from build123d import *

# Parameters (mm, degrees)
PAD_DEPTH       = 2
CHAMFER_SIZE    = 1
FILLET_R        = 1
SKETCH002_W     = 1.2
SKETCH002_H     = 3
PAD001_DEPTH    = 4.5
CHAMFER001_SIZE = 0.2


with BuildPart() as part:
    # Sketch → Pad (new body)
    with BuildSketch(Plane.XY):
        Polygon((17.999992, 0), (17.999992, 10.3923), (8.999996, 15.58845), (0, 10.3923), (0, 0), (8.999996, -5.19615), align=None)
    extrude(amount=PAD_DEPTH)

    # Chamfer
    chamfer_edges = [part.edges().sort_by_distance(p)[0] for p in [
        (13.499994, -2.598075, 2),
        (4.499998, -2.598075, 2),
        (17.999992, 5.19615, 2),
        (13.499994, 12.990375, 2),
        (0, 5.19615, 2),
        (4.499998, 12.990375, 2),
    ]]
    chamfer(chamfer_edges, length=CHAMFER_SIZE)

    # Fillet
    fillet_edges = [part.edges().sort_by_distance(p)[0] for p in [
        (13.499994, 12.990375, 1),
        (13.499994, -2.598075, 1),
        (17.999992, 5.19615, 1),
        (4.499998, -2.598075, 1),
        (0, 5.19615, 1),
        (4.499998, 12.990375, 1),
    ]]
    fillet(fillet_edges, radius=FILLET_R)

    # Sketch002 → Pad001 (join)
    with BuildSketch(Plane(origin=(0, 0, 0.01), x_dir=(1, 0, 0), z_dir=(0, 0, -1))):
        with Locations((6.149996, -5.19615)):
            Rectangle(SKETCH002_W, SKETCH002_H)
        with Locations((11.849996, -5.19615)):
            Rectangle(SKETCH002_W, SKETCH002_H)
    extrude(amount=PAD001_DEPTH)

    # Chamfer001
    chamfer001_edges = [part.edges().sort_by_distance(p)[0] for p in [
        (11.849996, 3.69615, -4.49),
        (11.249996, 5.19615, -4.49),
        (11.849996, 6.69615, -4.49),
        (12.449996, 5.19615, -4.49),
        (11.249996, 3.69615, -2.245),
        (11.249996, 6.69615, -2.245),
        (12.449996, 3.69615, -2.245),
        (12.449996, 6.69615, -2.245),
        (5.549996, 5.19615, -4.49),
        (6.149996, 3.69615, -4.49),
        (6.749996, 5.19615, -4.49),
        (6.149996, 6.69615, -4.49),
        (5.549996, 3.69615, -2.245),
        (6.749996, 3.69615, -2.245),
        (5.549996, 6.69615, -2.245),
        (6.749996, 6.69615, -2.245),
    ]]
    chamfer(chamfer001_edges, length=CHAMFER001_SIZE)


solid = part.part
Verification items for the finished model (mm, model axes). A direction names the side the tool comes from. Give positions to 0.01 mm unless a question says otherwise; leave off trailing zeros. Loops run counter-clockwise (first coordinate to the right, second up) from the corner with the lowest first, then second, coordinate; pieces in that order, holes last.
1) Sectioned sample at D-D, the plane z = 1. Enter the section's corners in (x, y).
2) Draft check along X on faces 6 (the flat face through (6, 5, -4.49)), 7 (the flat face through (5.55, 5, -2)), 8 (the flat face through (6.75, 5, -2)), 9 (the flat face through (13.563, 12.954, 0.289)). Enter one of: pulls with the +X half, pulls with the -X half, needs draft (parallel to the pull), parting line crosses it, or undercut.
3) Depth check by flat-ended pin: pin 1 Ø0.8 at (y, z) = (5, -2.5) entering from -X; pin 2 Ø6 at (x, y) = (13.5, 0.5) entering from -Z; pin 3 Ø0.9 at (x, z) = (6, -3) entering from -Y. Enter the tip coordinate at first touch or a pass-through.
4) Sectioned sample at C-C, the plane y = 7.25. Enter the section's corners in (x, z), then the cut area to 3 significant figures.
5) Sectioned sample at B-B, the plane y = 4.75. Enter the section's corners in (x, z).
6) Thickness scan on line 1 along Z through (x, y) = (12.75, 5.5); line 2 along Y through (x, z) = (13, 1); line 3 along Y through (x, z) = (1.5, 1.25). Record the ranges inside material, lowest first.
7) Set-up check for faces 1 (the flat face through (12, 6.696, -2)), 2 (the flat face through (12.45, 5, -2)), 3 (the flat face through (11.25, 5, -2)), 4 (the flat face through (12, 3.696, -2)), 5 (the flat face through (12, 5, -4.49)): record each of +Z, -Z, +X, -X, +Y, -Y from which the full face is reachable in a straight line by a thin tool's end or side.
8) Sectioned sample at A-A, the plane z = -0.75. Enter the section's corners in (x, y).
Answers:
1. outline: (0.09, 0.05) - (9, -5.09) - (17.91, 0.05) - (17.91, 10.34) - (9, 15.48) - (0.09, 10.34) - close
2. face 6: needs draft
2. face 7: pulls with the -X half
2. face 8: undercut
2. face 9: pulls with the +X half
3. pin 1: stops at x = 5.55
3. pin 2: stops at z = 0
3. pin 3: stops at y = 3.7
4. outline: (0, 0) - (18, 0) - (18, 0.59) arc R1 ccw to (17.71, 1.29) - (17, 2) - (1, 2) - (0.29, 1.29) arc R1 ccw to (0, 0.59) - close
4. area: 35.0 mm2
5. outline: (0, 0) - (5.55, 0) - (5.55, -4.29) - (5.75, -4.49) - (6.55, -4.49) - (6.75, -4.29) - (6.75, 0) - (11.25, 0) - (11.25, -4.29) - (11.45, -4.49) - (12.25, -4.49) - (12.45, -4.29) - (12.45, 0) - (18, 0) - (18, 0.59) arc R1 ccw to (17.71, 1.29) - (17, 2) - (1, 2) - (0.29, 1.29) arc R1 ccw to (0, 0.59) - close
6. line 1: z = 0 to 2
6. line 2: y = -2.78 to 13.18
6. line 3: y = -0.57 to 10.97
7. face 1: -Z, +X, -X, +Y
7. face 2: -Z, +X, +Y, -Y
7. face 3: -Z, +Y, -Y
7. face 4: -Z, +X, -X, -Y
7. face 5: -Z, +X, -X, +Y, -Y
8. outline: (5.55, 3.9) - (5.75, 3.7) - (6.55, 3.7) - (6.75, 3.9) - (6.75, 6.5) - (6.55, 6.7) - (5.75, 6.7) - (5.55, 6.5) - close; (11.25, 3.9) - (11.45, 3.7) - (12.25, 3.7) - (12.45, 3.9) - (12.45, 6.5) - (12.25, 6.7) - (11.45, 6.7) - (11.25, 6.5) - close
